```python
from build123d import *

# Parameters (mm, degrees)
F1_DEPTH = 25.4
F2_R     = 4.7625
F3_DEPTH = 25.4
F5_R     = 4.7625
F6_DEPTH = 9.525


with BuildPart() as f1:
    # F0 (on Right) → F1 (new body, symmetric)
    with BuildSketch(Plane.YZ):
        Polygon((310.379616, 9.525), (-19.820384, 9.525), (-19.820384, -9.525), (361.179616, -9.525), (361.179616, 0), (310.379616, 0), align=None)
    extrude(amount=F1_DEPTH, both=True)

    # F2 (on Top) → F3 (cut)
    with BuildSketch(Plane.XY):
        with Locations((0, 335.779616)):
            Circle(F2_R)
    extrude(amount=-F3_DEPTH, mode=Mode.SUBTRACT)

    # F5 (on offset) → F6 (join)
    with BuildSketch(Plane.XZ.offset(19.05)):
        Circle(F5_R)
    extrude(amount=F6_DEPTH)


solid = f1.part
```
Geometry check sheet. Reference: the model listing, model coordinates, mm. A direction names the side the tool comes from. Give positions to 0.01 mm unless a question says otherwise; leave off trailing zeros. Order: outer loops, then holes, each group sorted by start corner. A loop starts at its lowest first (then second) coordinate and runs counter-clockwise, first axis right, second up. Notation, with made-up numbers: (35, -29) - (39, -29) arc R17 ccw to (39, -21) - close; hole circle Ø9 at (15, -38). An arc over 180 degrees is marked (long way). Write item = value, one per line. Start each with the question number.
1) Draft check along X on faces 1 (the cylindrical face through (-0.62, 340.5, -4.7)), 2 (the flat face through (25.4, 168, 0)), 3 (the flat face through (0, 310.38, 5)). Enter one of: released by +X, released by -X, zero draft, split by the parting line, or undercut.
2) Section check A-A (x = 0). Enter the section's corners in (y, z) (1 decimal), then the cut area to 3 significant figures.
3) Section check B-B (x = -20.5). Enter the section's corners in (y, z) (3 decimals), then the cut area to 3 significant figures.
4) Gauge pin test, flat ends, axial feed: pin 1 Ø6 at (x, z) = (-7.5, 6) entering from -Y; pin 2 Ø4 at (x, y) = (-11, 313.5) entering from +Z; pin 3 Ø3 at (x, z) = (3, 3) entering from +Y. Record the tip position at first contact, or that the pin passes through.
5) Scan lines: L1, parallel to Y at x = 0, z = -6; L2, parallel to Y at x = 0, z = -1.75 (3 decimals); L3, parallel to Z at x = 1.5, y = 346 (3 decimals). Record each from-to range of solid material in increasing order.
6) Access from +Z, -Z, +X, -X, +Y, -Y to the whole of each face (thin tool, end or side, straight path). Record for faces 4 (the flat face through (0, 342, 0)), 5 (the flat face through (0, -28.575, 0)), 6 (the cylindrical face through (-3.78, -24.14, -2.9)).
Geometry check:
q1.face_1 = undercut
q1.face_2 = released by +X
q1.face_3 = zero draft
q2.outline = (-28.6, -4.8) - (-19.8, -4.8) - (-19.8, -9.5) - (331, -9.5) - (331, 0) - (310.4, 0) - (310.4, 9.5) - (-19.8, 9.5) - (-19.8, 4.8) - (-28.6, 4.8) - close; (340.5, -9.5) - (361.2, -9.5) - (361.2, 0) - (340.5, 0) - close
q2.area = 6,770 mm2
q3.outline = (-19.82, -9.525) - (361.18, -9.525) - (361.18, 0) - (310.38, 0) - (310.38, 9.525) - (-19.82, 9.525) - close
q3.area = 6,770 mm2
q4.pin_1 = -19.82
q4.pin_2 = 0
q4.pin_3 = 310.38
q5.L1 = -19.82 to 331.02, 340.54 to 361.18
q5.L2 = -28.575 to 331.017, 340.542 to 361.18
q5.L3 = -9.525 to 0
q6.face_4 = +Z, +X, -X, +Y
q6.face_5 = +Z, -Z, +X, -X, -Y
q6.face_6 = -Y
